Input: part model. Units: mm. Frame: model coordinates. A direction names the side the tool comes from. Round coordinates to 2 decimals unless told otherwise and drop trailing zeros. Loops run counter-clockwise (first coordinate to the right, second up) from the corner with the lowest first, then second, coordinate; pieces in that order, holes last. Notation, with made-up numbers: (33.25, 1.25) -> (83.25, 1.25) arc R22 ccw to (83.25, 37.25) -> close; hole circle Ø2 at (16.25, 14.25). An arc over 180 degrees is marked (long way). One line per question, with ' | ' between items. Start each with the question number.
Q1. Mould query, pull axis Y, two halves, no side actions, for faces 4 (the face through (3, 20, -20)), 5 (the face through (0, 0, -39)), 6 (the face through (14, 4.1, -6)). Classes: pulls with the +Y half, pulls with the -Y half, needs draft (parallel to the pull), parting line crosses it, or undercut.
Q2. Cut plane C-C on z = -7. Return loops of the section in (x, y), and give its area (3 significant figures).
Q3. Material intervals for L1, parallel to Y at x = 3, z = -55.75; L2, parallel to Y at x = 2.2, z = -42; L3, parallel to Z at x = 0.95, y = 13.5, sorted ascending.
Q4. Cut plane A-A on x = 17. Return loops of the section in (y, z), and give its area (3 significant figures).
Q5. Access query for faces 1 (the face through (1.479, 15.688, -76.696)), 2 (the face through (11, 14, 3)), 3 (the face through (6.46, -9.13, -44.44)). Directions: +Z, -Z, +X, -X, +Y, -Y. A direction counts if a zero-diameter tool reaches every point of the face in a straight line with its end or side. Return the directions, or none.
Q6. Cut plane B-B on y = 13. State how many separate pieces and enclosed holes the cut face has, and give its area (3 significant figures).
Q7. Contact query for flat-ended pins moving along their axis: P1, Ø1.3, axis at x = 22.1, y = 2, coming from the -Z side; P2, Ø10, axis at x = 22.5, y = -13.5, coming from the +Z side; P3, Ø5, axis at x = 16, y = 10, coming from the -Z side; P4, Ø6.5, axis at x = 19, y = 0.5, coming from the -Z side. Output: stop coordinate, or through.
Q8. Cut plane D-D on z = -38. Return loops of the section in (x, y), and give its area (3 significant figures).
from build123d import *

# Parameters (mm, degrees)
PAD008_DEPTH    = 4
PAD009_DEPTH    = 22.2
SKETCH_R        = 2
SKETCH_R_2      = 1.5
POCKET_DEPTH    = 26.201
SKETCH016_W     = 20.2
SKETCH016_H     = 20.2
POCKET001_DEPTH = 8
SKETCH017_R     = 1.1
SKETCH017_R_2   = 8.5
POCKET002_DEPTH = 50
SKETCH018_W     = 5.9
SKETCH018_H     = 13
POCKET003_DEPTH = 6.5
SKETCH019_W     = 3
SKETCH019_H     = 13
POCKET004_DEPTH = 5.501
SKETCH020_W     = 3
SKETCH020_H     = 13
POCKET005_DEPTH = 40
SKETCH021_R     = 5
POCKET006_DEPTH = 3
FILLET_R        = 6
SKETCH022_R     = 2.5
SKETCH022_R_2   = 1.5
PAD_DEPTH       = 5
CHAMFER_SIZE2   = 3
CHAMFER_SIZE    = 6


with BuildPart() as part:
    # Sketch013 → Pad008 (new body)
    with BuildSketch(Plane.YZ):
        Polygon((20, -89.25), (-20, -89.25), (-20, 0), (8, 0), (8, 10), (20, 10), align=None)
    extrude(amount=PAD008_DEPTH)

    # Sketch015 (on Face8 of Pad008) → Pad009 (join)
    with BuildSketch(Plane.YZ.offset(4)):
        Polygon((20, 10), (8, 10), (8, 0), (-20, 0), (-20, -10), (20, -10), align=None)
    extrude(amount=PAD009_DEPTH)

    # Sketch (on Face4 of Pad009) → Pocket (cut, through all)
    with BuildSketch(Plane(origin=(0, 0, 0), x_dir=(0, 1, 0), z_dir=(-1, 0, 0))):
        with Locations((-13.5, 82.75)):
            Circle(SKETCH_R)
        with Locations((13.5, 82.75)):
            Circle(SKETCH_R)
        with Locations((13.5, 55.75)):
            Circle(SKETCH_R)
        with Locations((-13.5, 55.75)):
            Circle(SKETCH_R)
        with Locations((13, 72.48)):
            Circle(SKETCH_R_2)
        with Locations((-8.59, 42)):
            Circle(SKETCH_R_2)
    extrude(amount=-POCKET_DEPTH, mode=Mode.SUBTRACT)

    # Sketch016 (on Face17 of Pocket) → Pocket001 (cut)
    with BuildSketch(Plane.YX.offset(10)):
        with Locations((-6, 14.1)):
            Rectangle(SKETCH016_W, SKETCH016_H)
    extrude(amount=-POCKET001_DEPTH, mode=Mode.SUBTRACT)

    # Sketch017 (on Face19 of Pocket001) → Pocket002 (cut)
    with BuildSketch(Plane(origin=(0, 0, 10), x_dir=(0, -1, 0), z_dir=(0, 0, 1))):
        with Locations((-2, 6.1)):
            Circle(SKETCH017_R)
        with Locations((14, 6.1)):
            Circle(SKETCH017_R)
        with Locations((14, 22.1)):
            Circle(SKETCH017_R)
        with Locations((-2, 22.1)):
            Circle(SKETCH017_R)
        with Locations((6, 14.1)):
            Circle(SKETCH017_R_2)
    extrude(amount=-POCKET002_DEPTH, mode=Mode.SUBTRACT)

    # Sketch018 (on Face22 of Pocket002) → Pocket003 (cut)
    with BuildSketch(Plane(origin=(0, 8, 0), x_dir=(0, 0, -1), z_dir=(0, -1, 0))):
        with Locations((-4.95, 17.5)):
            Rectangle(SKETCH018_W, SKETCH018_H)
    extrude(amount=-POCKET003_DEPTH, mode=Mode.SUBTRACT)

    # Sketch019 (on Face36 of Pocket003) → Pocket004 (cut, through all)
    with BuildSketch(Plane(origin=(0, 14.5, 0), x_dir=(0, 0, -1), z_dir=(0, -1, 0))):
        with Locations((-4.95, 17.5)):
            Rectangle(SKETCH019_W, SKETCH019_H)
    extrude(amount=-POCKET004_DEPTH, mode=Mode.SUBTRACT)

    # Sketch020 (on Face23 of Pocket004) → Pocket005 (cut)
    with BuildSketch(Plane(origin=(0, 0, 3.45), x_dir=(0, -1, 0), z_dir=(0, 0, 1))):
        with Locations((-17.5, 17.5)):
            Rectangle(SKETCH020_W, SKETCH020_H)
    extrude(amount=-POCKET005_DEPTH, mode=Mode.SUBTRACT)

    # Sketch021 (on Face4 of Pocket005) → Pocket006 (cut)
    with BuildSketch(Plane(origin=(0, 0, 0), x_dir=(0, 1, 0), z_dir=(-1, 0, 0))):
        with Locations((-8.59, 42)):
            Circle(SKETCH021_R)
        with Locations((13, 72.48)):
            Circle(SKETCH021_R)
    extrude(amount=-POCKET006_DEPTH, mode=Mode.SUBTRACT)

    # Fillet
    fillet_edges = [part.edges().sort_by_distance(p)[0] for p in [
        (2, -20, -89.25),
        (2, 20, -89.25),
    ]]
    fillet(fillet_edges, radius=FILLET_R)

    # Sketch022 → Pad (join)
    with BuildSketch(Plane.YZ.offset(4)):
        with Locations((-8.59, -42)):
            Circle(SKETCH022_R)
        with Locations((-8.59, -42)):
            Circle(SKETCH022_R_2, mode=Mode.SUBTRACT)
        with Locations((13, -72.48)):
            Circle(SKETCH022_R)
        with Locations((13, -72.48)):
            Circle(SKETCH022_R_2, mode=Mode.SUBTRACT)
    extrude(amount=PAD_DEPTH)

    # Chamfer
    chamfer_edges = [part.edges().sort_by_distance(p)[0] for p in [
        (0, 8, 5),
    ]]
    chamfer_side = part.faces().sort_by_distance((0, 0.384644, -41.786068))[0]
    chamfer(chamfer_edges, length=CHAMFER_SIZE, length2=CHAMFER_SIZE2, reference=chamfer_side)


solid = part.part
Results:
1) face 4: pulls with the +Y half | face 5: needs draft | face 6: undercut
2) outline: (0, -20) -> (26.2, -20) -> (26.2, 20) -> (0, 20) -> close; hole (4, -16.1) -> (24.2, -16.1) -> (24.2, 4.1) -> (4, 4.1) -> close; hole (11, 16) -> (24, 16) -> (24, 19) -> (11, 19) -> close | area: 601 mm^2
3) L1: -20 to -15.5, -11.5 to 11.5, 15.5 to 20 | L2: -20 to -13.59, -3.59 to 20 | L3: -89.25 to -84.75, -80.75 to -77.45, -67.51 to -57.75, -53.75 to 10
4) outline: (-20, -10) -> (-16.1, -10) -> (-16.1, -2) -> (-13.99, -2) -> (-13.99, 0) -> (-20, 0) -> close; (1.99, -2) -> (4.1, -2) -> (4.1, -10) -> (16, -10) -> (16, 3.45) -> (14.5, 3.45) -> (14.5, 2) -> (8, 2) -> (8, 0) -> (1.99, 0) -> close; (8, 7.9) -> (14.5, 7.9) -> (14.5, 6.45) -> (20, 6.45) -> (20, 10) -> (8, 10) -> close; (19, -10) -> (20, -10) -> (20, 3.45) -> (19, 3.45) -> close | area: 231 mm^2
5) face 1: -X | face 2: none | face 3: +X
6) separate pieces: 4 | enclosed holes: 1 | area: 705 mm^2
7) P1: through | P2: z = 0 | P3: z = -10 | P4: z = -2
8) outline: (0, -20) -> (4, -20) -> (4, 20) -> (0, 20) -> (0, -5.59) -> (3, -5.59) -> (3, -11.59) -> (0, -11.59) -> close | area: 142 mm^2
